Autodesk Fusion 360 part; units mm, degrees
sketch "Base_Sketch" plane through (0, 0, 0) normal (0, 0, 1) x (1, 0, 0)
  line L0 (57, 32) -> (-57, 32)
  line L1 (-57, -32) -> (57, -32)
  circle A0 centre (-57, 0) radius 11
  circle A1 centre (57, 0) radius 11
  arc A2 (-57, 32) -> (-57, -32) centre (-57, 0) ccw
  arc A3 (57, -32) -> (57, 32) centre (57, 0) ccw
  dimension "d1" = 114
  dimension "d2" = 64
  dimension "d3" = 32
  dimension "d4" = 32
extrude "Extrude1" add sketch "Base_Sketch" along normal blind 19
sketch "Top_Base_Sketch" plane through (0, 0, 19) normal (0, 0, 1) x (-1, 0, 0)
  circle A0 centre (-57, 0) radius 11
  circle A1 centre (57, 0) radius 11
  arc A2 (-57, 32) -> (-57, -32) centre (-57, 0) ccw
  line L0 (-57, -32) -> (57, -32)
  arc A3 (57, -32) -> (57, 32) centre (57, 0) ccw
  line L1 (57, 32) -> (-57, 32)
  line L2 (32, -32) -> (32, 32)
  line L3 (-32, -32) -> (-32, 32)
  line L4 (19, 32) -> (19, -19)
  line L5 (-18.7586, 32) -> (-18.7586, -19)
  line L6 (19, -19) -> (-19, -19)
  line L7 (32, 32) -> (19, 32) construction
  line L8 (32, -32) -> (-32, -32) construction
  line L9 (-18.7586, 32) -> (-32, 32) construction
  dimension "d9" = 64
  dimension "d11" = 51
  dimension "d12" = 51
  dimension "d13" = 38
  dimension "d15" = 13
extrude "Extrude2" add sketch "Top_Base_Sketch" along normal blind 45 contours L0 L1 L2 L3 L4 L5 L6
sketch "Triangle_Sketch" plane through (0, 0, 0) normal (1, 0, 0) x (0, 1, 0)
  line L0 (18.9506, 63.9102) -> (18.9506, 18.9102)
  line L1 (18.9506, 18.9102) -> (-32.0494, 18.9102)
  line L2 (-32.0494, 18.9102) -> (18.9506, 63.9102)
  dimension "d18" = 45
  dimension "d20" = 51
extrude "Extrude3" add sketch "Triangle_Sketch" along normal mid plane 38
The model under review builds one solid part; all positions refer to its coordinate system, in mm. A direction names the side the tool comes from. Round coordinates to 2 decimals unless told otherwise and drop trailing zeros. Order: outer loops, then holes, each group sorted by start corner. A loop starts at its lowest first (then second) coordinate and runs counter-clockwise, first axis right, second up. Notation, with made-up numbers: (5.5, 22.5) - (61.5, 22.5) arc R26 ccw to (61.5, 44.5) - close; hole circle Ø7 at (-26.75, 16.25). An arc over 180 degrees is marked (long way). Answer in a Markdown table with one row per item.
(1) Machinability: for faces 1 (the face through (88.992, 0.704, 9.367)), 2 (the face through (-32, 0, 41)), 3 (the face through (46, 0, 9)), 4 (the face through (-0.4, -6.9, 41.1)), 5 (the face through (66, 8, 19)), which of the approach directions +Z, -Z, +X, -X, +Y, -Y give a long, thin tool a straight path to every point of the face, cutting with its end or side? Answer none if there is none.
Result set:
| item | result |
|---|---|
| face 1 | +Z, -Z, +X |
| face 2 | +Z, -X, +Y, -Y |
| face 3 | +Z, -Z |
| face 4 | +Z, -Y |
| face 5 | +Z, +X, +Y, -Y |
(2) For line 1 (Y direction, x = -57, z = 12.25); line 2 (X direction, y = -29, z = 39.5); line 3 (Z direction, x = 62.5, y = 22), list the stretches that pass through material, from the lowest coordinate up. Write a range as from..to.
Result set:
| item | result |
|---|---|
| line 1 | y = -32..-11, 11..32 |
| line 2 | x = -32..-19, 18.76..32 |
| line 3 | z = 0..19 |
(3) Mouldability with a two-part tool opening along Y and no side actions: class faces 6 (the face through (-67, 8, 19)), 7 (the face through (1, 32, 24)), 8 (the face through (-68, 0, 9)) as released by +Y, released by -Y, zero draft, split by the parting line, or undercut.
Result set:
| item | result |
|---|---|
| face 6 | zero draft |
| face 7 | released by +Y |
| face 8 | undercut |
(4) Take a section at B-B on y = -8. Write out the cut boundary in (x, z).
Result set:
| item | result |
|---|---|
| outline | (-87.98, 0) - (-64.55, 0) - (-64.55, 19) - (-87.98, 19) - close; (-49.45, 0) - (49.45, 0) - (49.45, 19) - (32, 19) - (32, 64) - (18.76, 64) - (18.76, 40.13) - (-19, 40.13) - (-19, 64) - (-32, 64) - (-32, 19) - (-49.45, 19) - close; (64.55, 0) - (87.98, 0) - (87.98, 19) - (64.55, 19) - close |
(5) Take a section at A-A on x = 51. Write out the cut boundary in (y, z).
Result set:
| item | result |
|---|---|
| outline | (-32, 0) - (-9.22, 0) - (-9.22, 19) - (-32, 19) - close; (9.22, 0) - (32, 0) - (32, 19) - (9.22, 19) - close |
(6) Take a section at D-D on z = 34. Write out the cut boundary in (x, y), plus the area to 3 significant figures.
Result set:
| item | result |
|---|---|
| outline | (-32, -32) - (-19, -32) - (-19, -14.95) - (18.76, -14.95) - (18.76, -32) - (32, -32) - (32, 32) - (-32, 32) - close; hole (-19, 18.95) - (18.76, 18.95) - (18.76, 19) - (-19, 19) - close |
| area | 3,450 mm2 |
(7) Clearance check with flat-ended pins moving along their axes: P1, Ø3, axis at y = 3.5, z = 11.5, coming from the +X side; P2, Ø13.5, axis at y = -2.5, z = 51.5, coming from the +X side; P3, Ø17.5, axis at x = -57, y = 0, coming from the -Z side; P4, Ø17, axis at x = 50, y = -12.5, coming from the +Z side. State where each tip first meets the part, or that it passes through.
Result set:
| item | result |
|---|---|
| P1 | stops at x = 88.94 |
| P2 | stops at x = 32 |
| P3 | passes through |
| P4 | stops at z = 19 |
(8) Take a section at C-C on z = 14. Write out the cut boundary in (x, y), plus the area to 3 significant figures.
Result set:
| item | result |
|---|---|
| outline | (-57, -32) - (57, -32) arc R32 ccw to (57, 32) - (-57, 32) arc R32 ccw to start; hole circle Ø22 at (-57, 0); hole circle Ø22 at (57, 0) |
| area | 9,750 mm2 |
